Source: three-view drawing plus pictorial views. Frame: mm from the lowest corner of the part. A direction names the side the tool comes from. Give positions to 0.01 mm unless a question says otherwise; leave off trailing zeros. Write each loop counter-clockwise with the first axis right and the second up, starting at its lowest first coordinate (ties: lowest second). Pieces come first, ordered by that corner, then holes. Notation, with made-up numbers: (37, -7.5) -> (76, -7.5) arc R26 cw to (76, 22.5) -> close; hole circle Ø10 at (57.25, 8). An arc over 180 degrees is marked (long way). Write item = value, one per line.
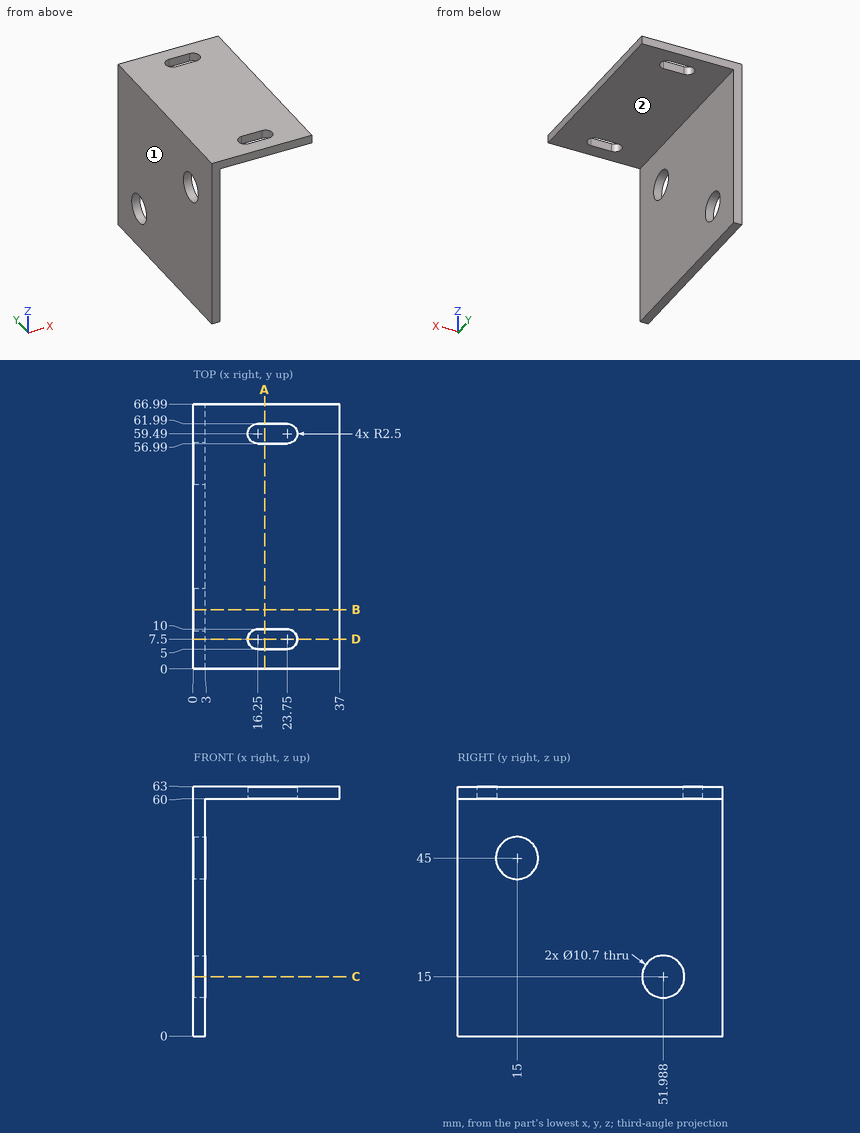
1) Access query for the marked faces 1 and 2. Directions: +Z, -Z, +X, -X, +Y, -Y. A direction counts if a zero-diameter tool reaches every point of the face in a straight line with its end or side. Return the directions, or none.
Computed:
face_1 = +Z, -Z, -X, +Y, -Y
face_2 = -Z, +X, +Y, -Y
2) Cut plane D-D (y = 7.5). Return the cut outline in (x, z).
Computed:
outline = (0, 0) -> (3, 0) -> (3, 60) -> (13.75, 60) -> (13.75, 63) -> (0, 63) -> close; (26.25, 60) -> (37, 60) -> (37, 63) -> (26.25, 63) -> close
3) Cut plane A-A (x = 18). Return the cut outline in (y, z), then the cut area to 3 significant figures.
Computed:
outline = (0, 60) -> (5, 60) -> (5, 63) -> (0, 63) -> close; (10, 60) -> (56.99, 60) -> (56.99, 63) -> (10, 63) -> close; (61.99, 60) -> (66.99, 60) -> (66.99, 63) -> (61.99, 63) -> close
area = 171 mm²
4) Material intervals for L1, parallel to Y at x = 1.4, z = 45; L2, parallel to Y at x = 2.1, z = 15; L3, parallel to Z at x = 7, y = 33.5, sorted ascending.
Computed:
L1 = 0 to 9.65, 20.35 to 66.99
L2 = 0 to 46.64, 57.34 to 66.99
L3 = 60 to 63
5) Cut plane C-C (z = 15). Return the cut outline in (x, y).
Computed:
outline = (0, 0) -> (3, 0) -> (3, 46.64) -> (0, 46.64) -> close; (0, 57.34) -> (3, 57.34) -> (3, 66.99) -> (0, 66.99) -> close
6) Contact query for flat-ended pins moving along their axis: pin 1 (3 mm diameter, centred on x = 9.5, y = 31.5, fed in from -Z); pin 2 (0.9 mm diameter, centred on x = 21.5, z = 62, fed in from -Y); pin 3 (10 mm diameter, centred on y = 34.5, z = 21.5, fed in from +X). Output: stop coordinate, or through.
Computed:
pin_1 = 60
pin_2 = 0
pin_3 = 3
7) Cut plane B-B (y = 15). Return the cut outline in (x, z), then the cut area to 3 significant figures.
Computed:
outline = (0, 0) -> (3, 0) -> (3, 39.65) -> (0, 39.65) -> close; (0, 50.35) -> (3, 50.35) -> (3, 60) -> (37, 60) -> (37, 63) -> (0, 63) -> close
area = 259 mm²
